Autodesk Inventor part; units mm, degrees
ref_plane "YZ Plane" through (0, 0, 0) normal (1, 0, 0) x (0, 1, 0)
ref_plane "XZ Plane" through (0, 0, 0) normal (0, 1, 0) x (-1, 0, 0)
ref_plane "XY Plane" through (0, 0, 0) normal (0, 0, 1) x (1, 0, 0)
sketch "Sketch1" plane through (0, 0, 0) normal (0, 1, 0) x (-1, 0, 0)
  line L0 (0, 0) -> (-12.5, 0)
  line L1 (0, 0) -> (12.5, 0)
  line L2 (12.5, 0) -> (12.5, -30)
  line L3 (-12.5, 0) -> (-12.5, -30)
  line L4 (12.5, -30) -> (17.5, -30)
  line L5 (17.5, -30) -> (17.5, 5)
  line L6 (-12.5, -30) -> (-17.5, -30)
  line L7 (-17.5, -30) -> (-17.5, 5)
  line L8 (-17.5, 5) -> (17.5, 5)
  dimension "d0" = 12.5
  dimension "d1" = 12.5
  dimension "d2" = 30
  dimension "d3" = 30
  dimension "d4" = 5
  dimension "d5" = 35
  dimension "d6" = 5
  dimension "d7" = 35
extrude "Extrusion1" add sketch "Sketch1" along normal blind 10
sketch "Sketch2" plane through (17.5, 0, 5) normal (1, 0, 0) x (0, 0, -1)
  line L0 (35, 0) -> (35, 10)
  line L1 (35, 5) -> (25, 5)
  circle A0 centre (25, 5) radius 2.5
  point P0 (5, 0)
  dimension "d10" = 10
  dimension "d11" = 5
extrude "Extrusion2" cut sketch "Sketch2" against normal blind 35
sketch "Sketch3" plane through (-17.5, 0, 5) normal (0, 0, 1) x (1, 0, 0)
  line L0 (5, 10) -> (0, 10)
  line L1 (30, 0) -> (35, 0)
  line L2 (0, 10) -> (35, 0)
  circle A0 centre (17.5, 5) radius 4
  circle A1 centre (17.5, 5) radius 2.5
  point P0 (17.5, 0)
  dimension "d14" = 8
  dimension "d15" = 5
extrude "Extrusion3" add sketch "Sketch3" along normal blind 10 contours A0 L2 A1 | L2 A1 A0
properties part number "BaseFork"
Here's how the part is built. I have some questions about the finished solid (model axes, mm). A direction names the side the tool comes from. Give positions to 0.01 mm unless a question says otherwise; leave off trailing zeros. Order: outer loops, then holes, each group sorted by start corner. A loop starts at its lowest first (then second) coordinate and runs counter-clockwise, first axis right, second up. Notation, with made-up numbers: (-31, 79.25) -> (-8, 79.25) arc R13 ccw to (-8, 83.25) -> close; hole circle Ø5 at (25, 67.5). An arc over 180 degrees is marked (long way). Use CSV: the item, a comma, the result in double quotes. Start each with the question number.
Item 1: If I drill on probe 1 along X at (y, z) = (8.5, -27); probe 2 along Y at (x, z) = (-16.35, -20); probe 3 along Z at (x, y) = (-11.5, 8.25), over which ranges is the centre line in solid material (lowest first)? Write a range as [from, to].
Item 2: Suppose I cut it at B-B (y = 5). List the corners of the cut face in (x, z) for me, and give its area (3 significant figures).
Item 3: I'm going to push flat-ended pins straight in: P1, Ø6, axis at y = 5, z = -20, coming from the +X side; P2, Ø1, axis at x = -3, y = 9, coming from the -Z side; P3, Ø4, axis at x = -6.5, y = 2.5, coming from the +Z side. Where does each tip first touch, or does it pass through?
Item 4: Suppose I cut it at C-C (x = 14). List the corners of the cut face in (y, z) for me.
Item 5: On a 3-axis mill with a long thin cutter (end or side, diameter ignored), from which of +Z, -Z, +X, -X, +Y, -Y can I reach the whole of each face in a straight line? I mean faces 4 (the flat face through (-12.5, 5, -15)), 5 (the flat face through (0, 5, 5)), 6 (the flat face through (-15, 5, -30)). Say none if no direction works.
Item 6: Suppose I cut it at A-A (z = -7.5). List the corners of the cut face in (x, y) for me.
Item 7: Thinking about a two-plate mould opening in Z: for faces 1 (the flat face through (0, 5, 0)), 2 (the flat face through (4.1, 6, 5)), 3 (the cylindrical face through (15, 5.1, -17.5)), which applies, pulls with the +Z half, pulls with the -Z half, needs draft (parallel to the pull), parting line crosses it, or undercut?
Item 8: Suppose I cut it at D-D (z = -20). List the corners of the cut face in (x, y) for me, and give its area (3 significant figures).
Answer block:
1,probe 1,"x = [-17.5, -12.5], [12.5, 17.5]"
1,probe 2,"y = [0, 2.5], [7.5, 10]"
1,probe 3,"z = [0, 5]"
2,outline,"(-17.5, -30) -> (-12.5, -30) -> (-12.5, -22.5) -> (-17.5, -22.5) -> close; (-17.5, -17.5) -> (-12.5, -17.5) -> (-12.5, 0) -> (12.5, 0) -> (12.5, -17.5) -> (17.5, -17.5) -> (17.5, 5) -> (4, 5) -> (4, 15) -> (2.5, 15) -> (2.5, 5) -> (-2.5, 5) -> (-2.5, 15) -> (-4, 15) -> (-4, 5) -> (-17.5, 5) -> close; (12.5, -30) -> (17.5, -30) -> (17.5, -22.5) -> (12.5, -22.5) -> close"
2,area,"455 mm^2"
3,P1,"stops at x = 17.5"
3,P2,"stops at z = 0"
3,P3,"stops at z = 5"
4,outline,"(0, -30) -> (10, -30) -> (10, 5) -> (0, 5) -> close; hole circle Ø5 at (5, -20)"
5,face 4,"-Z, +Y, -Y"
5,face 5,"+Z"
5,face 6,"-Z, +X, -X, +Y, -Y"
6,outline,"(-17.5, 0) -> (-12.5, 0) -> (-12.5, 10) -> (-17.5, 10) -> close; (12.5, 0) -> (17.5, 0) -> (17.5, 10) -> (12.5, 10) -> close"
7,face 1,"pulls with the -Z half"
7,face 2,"pulls with the +Z half"
7,face 3,"undercut"
8,outline,"(-17.5, 0) -> (-12.5, 0) -> (-12.5, 2.5) -> (-17.5, 2.5) -> close; (-17.5, 7.5) -> (-12.5, 7.5) -> (-12.5, 10) -> (-17.5, 10) -> close; (12.5, 0) -> (17.5, 0) -> (17.5, 2.5) -> (12.5, 2.5) -> close; (12.5, 7.5) -> (17.5, 7.5) -> (17.5, 10) -> (12.5, 10) -> close"
8,area,"50.0 mm^2"
